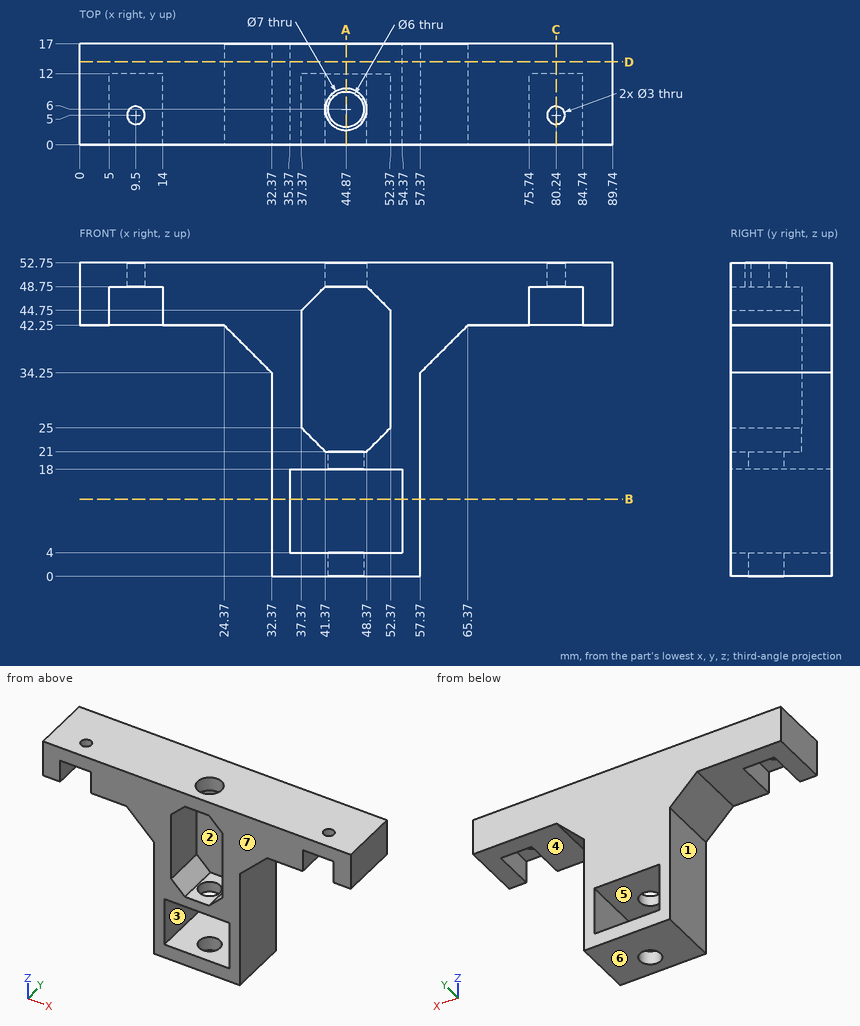
Design review of the part shown in the three views and the two pictorial views. Dimensions are in mm from the part's minimum x, y and z. A direction names the side the tool comes from. Give positions to 0.01 mm unless a question says otherwise; leave off trailing zeros. Loops run counter-clockwise (first coordinate to the right, second up) from the corner with the lowest first, then second, coordinate; pieces in that order, holes last. Notation, with made-up numbers: (42.5, 18) - (50.5, 18) arc R19 ccw to (50.5, 24) - close; hole circle Ø9 at (-16, 49.5). An arc over 180 degrees is marked (long way). Answer as a JSON object with one key per item and string values.
Q1. Add section D-D on y = 14. State the section outline as (x, z) points.
Worked out:
{"outline": "(0, 42.25) - (24.37, 42.25) - (32.37, 34.25) - (32.37, 0) - (57.37, 0) - (57.37, 34.25) - (65.37, 42.25) - (89.74, 42.25) - (89.74, 52.75) - (0, 52.75) - close; hole (35.37, 4) - (54.37, 4) - (54.37, 18) - (35.37, 18) - close"}
Q2. To check wall thickness, follow line 1 along Y through (x, z) = (44.87, 1.55); line 2 along X through (y, z) = (11, 8); line 3 along Z through (x, y) = (45, 9.25). State the ranges of each line that lie inside material, in increasing order.
Worked out:
{"line 1": "y = 0 to 3, 9 to 17", "line 2": "x = 32.37 to 35.37, 54.37 to 57.37", "line 3": "z = 0 to 4, 18 to 21"}
Q3. Mouldability with a two-part tool opening along Z and no side actions: class the marked faces 5, 6 and 7 as +Z half, -Z half, draft (parallel to the pull), parting line (faces both ways), or undercut.
Worked out:
{"face 5": "undercut", "face 6": "-Z half", "face 7": "draft"}
Q4. Add section C-C on x = 80.24. State the section outline as (y, z) points.
Worked out:
{"outline": "(0, 48.75) - (3.5, 48.75) - (3.5, 52.75) - (0, 52.75) - close; (6.5, 48.75) - (12, 48.75) - (12, 42.25) - (17, 42.25) - (17, 52.75) - (6.5, 52.75) - close"}
Q5. Add section B-B on z = 13. State the section outline as (x, y) points.
Worked out:
{"outline": "(32.37, 0) - (35.37, 0) - (35.37, 17) - (32.37, 17) - close; (54.37, 0) - (57.37, 0) - (57.37, 17) - (54.37, 17) - close"}
Q6. Add section A-A on x = 44.87. State the section outline as (y, z) points.
Worked out:
{"outline": "(0, 0) - (3, 0) - (3, 4) - (0, 4) - close; (0, 18) - (3, 18) - (3, 21) - (0, 21) - close; (0, 48.75) - (2.5, 48.75) - (2.5, 52.75) - (0, 52.75) - close; (9, 0) - (17, 0) - (17, 4) - (9, 4) - close; (9, 18) - (17, 18) - (17, 52.75) - (9.5, 52.75) - (9.5, 48.75) - (12, 48.75) - (12, 21) - (9, 21) - close"}
Q7. Insertion check: pin 1 (3 mm diameter, centred on x = 8, z = 45, fed in from -Y); pin 2 (10 mm diameter, centred on x = 9.5, y = 5, fed in from -Z); pin 3 (8.5 mm diameter, centred on y = 12.5, z = 24, fed in from -X). Each pin has a flat end and moves straight along its axis. Give the tip position at first contact, or say it passes through.
Worked out:
{"pin 1": "stops at y = 12", "pin 2": "stops at z = 42.25", "pin 3": "stops at x = 32.37"}
Q8. For the marked faces 1, 2, 3 and 4, list the 3-axis set-ups (+Z, -Z, +X, -X, +Y, -Y) from which the entire face can be reached by the end or side of a thin tool; tool diameter is ignored.
Worked out:
{"face 1": "-Z, -X, +Y, -Y", "face 2": "-Y", "face 3": "+Y, -Y", "face 4": "-Z, +X, +Y, -Y"}
